Build history of the part. All positions in model axes, mm. A direction names the side the tool comes from. Round coordinates to 2 decimals unless told otherwise and drop trailing zeros. Loops run counter-clockwise (first coordinate to the right, second up) from the corner with the lowest first, then second, coordinate; pieces in that order, holes last. Notation, with made-up numbers: (-4.5, 8) -> (36.5, 8) arc R28 ccw to (36.5, 36) -> close; hole circle Ø2 at (53, 11.5). An arc over 180 degrees is marked (long way). Put each result on its own line as item: value. Start each with the question number.
Item 1: Drill centre lines: probe 1 along Y at (x, z) = (2.25, 2.45); probe 2 along Y at (x, z) = (2, 0.2); probe 3 along Y at (x, z) = (-0.5, 0.85). Where is each one in solid material? Low to high. Write a range as [from, to].
Item 2: Cut at C-C, the plane z = 1.7. List the corners of the cut face in (x, y) (3 decimals).
Item 3: Cut at A-A, the plane x = 0.5. List the corners of the cut face in (y, z).
Item 4: Pull direction Y, two halves, no side cores. Call faces 1 (the flat face through (-3.375, -7, 1)), 2 (the cylindrical face through (1.803, 2.853, 1.232)), 3 (the cylindrical face through (1.417, -13.414, 1.232)): +Y half, -Y half, draft (parallel to the pull), parting line (faces both ways), or undercut.
Item 5: Cut at D-D, the plane x = 3. List the corners of the cut face in (y, z).
Item 6: Cut at B-B, the plane y = -1. List the corners of the cut face in (x, z) (3 decimals), plus the area to 3 significant figures.
Item 7: Flat gauge pins, fed straight in: pin 1 Ø2.5 at (x, y) = (1.625, -15) entering from +Z; pin 2 Ø1 at (y, z) = (-17, 1.5) entering from +X. Where does each tip first touch, or does it go through?
Item 8: Tool access for faces 4 (the flat face through (0, -11, 2.5)), 5 (the flat face through (1.625, -7, 1)): list every direction of +Z, -Z, +X, -X, +Y, -Y with a clear straight run to the whole face (end or side of a thin tool).
```python
from build123d import *

# Parameters (mm, degrees)
SKETCH1_R           = 5
SKETCH1_R_2         = 1.6
SKETCH1_R_3         = 3.375
BOSS_EXTRUDE1_DEPTH = 2.5


with BuildPart() as part:
    # Sketch1 → Boss-Extrude1 (new body)
    with BuildSketch(Plane.XY):
        with Locations((1.625, -15)):
            Circle(SKETCH1_R)
        with Locations((1.625, -15)):
            Circle(SKETCH1_R_2, mode=Mode.SUBTRACT)
        with BuildLine():
            Line((-3.375, 0), (-3.375, -15))
            ThreePointArc((-3.375, -15), (-1.910533906, -11.464466094), (1.625, -10))
            Line((1.625, -10), (1.625, -2.958039892))
            ThreePointArc((1.625, -2.958039892), (-1.718465886, -2.90473751), (-3.375, 0))
        make_face()
        Circle(SKETCH1_R_3)
        Circle(SKETCH1_R_2, mode=Mode.SUBTRACT)
    extrude(amount=BOSS_EXTRUDE1_DEPTH)


solid = part.part
```
Reply:
1. probe 1: y = [-19.96, -16.47], [-13.53, -10.04], [-2.52, 2.52]
1. probe 2: y = [-19.99, -16.56], [-13.44, -10.01], [-2.72, 2.72]
1. probe 3: y = [-19.53, -1.52], [1.52, 3.34]
2. outline: (-3.375, -15) arc R5 ccw (long way) to (1.625, -10) -> (1.625, -2.958) arc R3.375 ccw (long way) to (-3.375, 0) -> close; hole circle Ø3.2 at (0, 0); hole circle Ø3.2 at (1.625, -15)
3. outline: (-19.87, 0) -> (-16.14, 0) -> (-16.14, 2.5) -> (-19.87, 2.5) -> close; (-13.86, 0) -> (-1.52, 0) -> (-1.52, 2.5) -> (-13.86, 2.5) -> close; (1.52, 0) -> (3.34, 0) -> (3.34, 2.5) -> (1.52, 2.5) -> close
4. face 1: draft
4. face 2: undercut
4. face 3: undercut
5. outline: (-19.81, 0) -> (-15.82, 0) -> (-15.82, 2.5) -> (-19.81, 2.5) -> close; (-14.18, 0) -> (-10.19, 0) -> (-10.19, 2.5) -> (-14.18, 2.5) -> close; (-1.55, 0) -> (1.55, 0) -> (1.55, 2.5) -> (-1.55, 2.5) -> close
6. outline: (-3.375, 0) -> (-1.249, 0) -> (-1.249, 2.5) -> (-3.375, 2.5) -> close; (1.249, 0) -> (3.223, 0) -> (3.223, 2.5) -> (1.249, 2.5) -> close
6. area: 10.3 mm^2
7. pin 1: passes through
7. pin 2: stops at x = 6.39
8. face 4: +Z, +X, -X, +Y, -Y
8. face 5: +Z, -Z, +X
